Can you work these out from the model? Positions are in its coordinate system, mm. A direction names the side the tool comes from. Give positions to 0.01 mm unless a question says otherwise; leave off trailing zeros. Loops run counter-clockwise (first coordinate to the right, second up) from the corner with the lowest first, then second, coordinate; pieces in that order, holes last. Notation, with made-up numbers: (-17.75, 55) - (36.25, 55) arc R13 ccw to (36.25, 75) - close; hole circle Ø4 at (4, -13). An arc over 180 degrees is marked (long way). Answer in a Markdown table with one row per item.
from build123d import *

# Parameters (mm, degrees)
BASE_FLANGE1_DEPTH = 20.0914
SKETCH6_R          = 5.08
CUT_EXTRUDE1_DEPTH = 71.148762412
FILLET1_R          = 6.35
SKETCH7_R          = 2.4892
CUT_EXTRUDE2_DEPTH = 73.473753725


# Sheet-metal steps are written as plain solids
with BuildPart() as part:
    # Sketch1 → Base-Flange1 (new body)
    with BuildSketch(Plane(origin=(0, 0, 0), x_dir=(1, 0, 0), z_dir=(0, 1, 0))):
        with BuildLine():
            Line((0, -28.575), (0, -3.429))
            ThreePointArc((0, -3.429), (1.004330847, -1.004330847), (3.429, 0))
            Line((3.429, 0), (63.5, 0))
            Line((63.5, 0), (63.5, -2.667))
            Line((63.5, -2.667), (3.429, -2.667))
            ThreePointArc((3.429, -2.667), (2.890184633, -2.890184633), (2.667, -3.429))
            Line((2.667, -3.429), (2.667, -28.575))
            Line((2.667, -28.575), (0, -28.575))
        make_face()
    extrude(amount=BASE_FLANGE1_DEPTH)

    # Sketch6 → Cut-Extrude1 (cut, through all)
    with BuildSketch(Plane(origin=(2.667, 0, 0), x_dir=(0, 0, -1), z_dir=(1, 0, 0))):
        with Locations((-19.05, 10.0457)):
            Circle(SKETCH6_R)
    extrude(amount=-CUT_EXTRUDE1_DEPTH, mode=Mode.SUBTRACT)

    # Fillet1
    fillet1_edges = [part.edges().sort_by_distance(p)[0] for p in [
        (1.3335, 20.0914, 28.575),
        (1.3335, 0, 28.575),
        (63.5, 20.0914, 1.3335),
        (63.5, 0, 1.3335),
    ]]
    fillet(fillet1_edges, radius=FILLET1_R)

    # Sketch7 → Cut-Extrude2 (cut, through all)
    with BuildSketch(Plane(origin=(0, 0, 0), x_dir=(-1, 0, 0), z_dir=(0, 0, -1))):
        with Locations((-50.8, 10.0457)):
            Circle(SKETCH7_R)
        with Locations((-38.1, 10.0457)):
            Circle(SKETCH7_R)
        with Locations((-25.4, 10.0457)):
            Circle(SKETCH7_R)
        with Locations((-12.7, 10.0457)):
            Circle(SKETCH7_R)
    extrude(amount=-CUT_EXTRUDE2_DEPTH, mode=Mode.SUBTRACT)


solid = part.part
Q1. Imagine slicing it at D-D, the plane z = 6.75. Write out the boundary of the cut face in (x, y), and give its area (3 significant figures).
Checked values:
| item | result |
|---|---|
| outline | (0, 0) - (2.67, 0) - (2.67, 20.09) - (0, 20.09) - close |
| area | 53.6 mm² |
Q2. On a 3-axis mill with a long thin cutter (end or side, diameter ignored), from which of +Z, -Z, +X, -X, +Y, -Y can I reach the whole of each face in a straight line? I mean faces 1 (the face through (34, 10, 2.667)), 2 (the face through (63.5, 10, 1)). Say none if no direction works.
Checked values:
| item | result |
|---|---|
| face 1 | +Z, +X, +Y, -Y |
| face 2 | +Z, -Z, +X, +Y, -Y |
Q3. Imagine slicing it at B-B, the plane x = 38.1. Write out the boundary of the cut face in (y, z).
Checked values:
| item | result |
|---|---|
| outline | (0, 0) - (7.56, 0) - (7.56, 2.67) - (0, 2.67) - close; (12.53, 0) - (20.09, 0) - (20.09, 2.67) - (12.53, 2.67) - close |
Q4. Imagine slicing it at C-C, the plane y = 18.5. Write out the boundary of the cut face in (x, z).
Checked values:
| item | result |
|---|---|
| outline | (0, 3.43) arc R3.43 ccw to (3.43, 0) - (61.35, 0) - (61.35, 2.67) - (3.43, 2.67) arc R0.76 cw to (2.67, 3.43) - (2.67, 26.43) - (0, 26.43) - close |
Q5. For pin 1 (2 mm diameter, centred on x = 16.5, y = 12, fed in from +Z); pin 2 (10 mm diameter, centred on y = 13.5, z = 16.5, fed in from +X), each with a flat end and sliding along its axis, tell me the tip position at first contact or that it passes through.
Checked values:
| item | result |
|---|---|
| pin 1 | stops at z = 2.67 |
| pin 2 | stops at x = 2.67 |
Q6. If we mould it in two halves opening along X, with no side actions, what happens to faces 3 (the face through (11.55, 7.84, 1.31)), 4 (the face through (61.59, 18.28, 1.35)), 5 (the face through (1.315, 18.182, 26.764))? For each: released by +X, released by -X, zero draft, split by the parting line, or undercut.
Checked values:
| item | result |
|---|---|
| face 3 | undercut |
| face 4 | released by +X |
| face 5 | zero draft |
Q7. Imagine slicing it at A-A, the plane z = 19.05. Write out the boundary of the cut face in (x, y), and give its area (3 significant figures).
Checked values:
| item | result |
|---|---|
| outline | (0, 0) - (2.67, 0) - (2.67, 4.97) - (0, 4.97) - close; (0, 15.13) - (2.67, 15.13) - (2.67, 20.09) - (0, 20.09) - close |
| area | 26.5 mm² |
Q8. If I drill on line 1 (Y direction, x = 50.8, z = 1.15); line 2 (X direction, y = 8, z = 2.5); line 3 (Z direction, x = 58, y = 9.5), over which ranges is the centre line in solid material (lowest first)? Write a range as [from, to].
Checked values:
| item | result |
|---|---|
| line 1 | y = [0, 7.56], [12.53, 20.09] |
| line 2 | x = [0.13, 11.28], [14.12, 23.98], [26.82, 36.68], [39.52, 49.38], [52.22, 63.5] |
| line 3 | z = [0, 2.67] |
